Can you work these out from the model? Positions are in its coordinate system, mm. Face numbers are marked on the shaded views. Give positions to 0.01 mm unless a question says otherwise; leave off trailing zeros. Write each loop counter-clockwise with the first axis right and the second up, starting at its lowest first coordinate (ties: lowest second). Pieces come first, ordered by that corner, then holes. Notation, with made-up numbers: M 89.25,-11 L 136.25,-11 A17 cw 136.25,8 Z; hole C 9,55 d9. An arc over 180 degrees is marked long. Use CSV: the item, a comma, the result in double quotes. Start each with the question number.
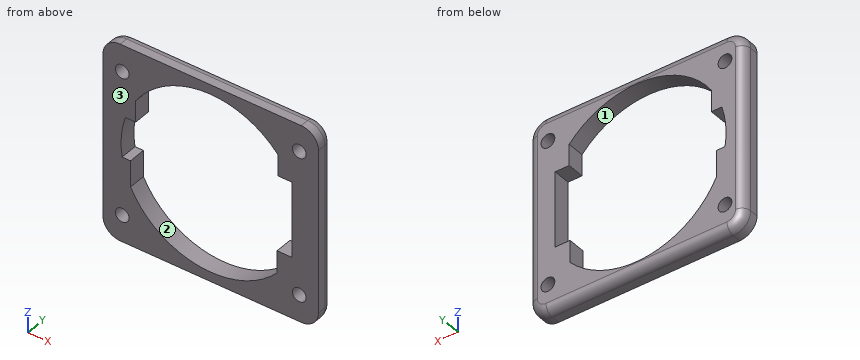
from build123d import *

# Parameters (mm, degrees)
SKETCH1_W           = 31.75
SKETCH1_H           = 29.21
BOSS_EXTRUDE1_DEPTH = 2.54
CUT_EXTRUDE1_DEPTH  = 22.720341848
SKETCH3_W           = 4.064
SKETCH3_H           = 4.263952617
SKETCH3_W_2         = 4.826
SKETCH3_H_2         = 10.541
SKETCH3_W_3         = 5.969
SKETCH3_H_3         = 4.464530762
SKETCH3_W_4         = 6.096
SKETCH3_H_4         = 4.639521707
BOSS_EXTRUDE2_DEPTH = 2.54
FILLET1_R           = 1.27
SKETCH5_R           = 1.016
CUT_EXTRUDE3_DEPTH  = 22.720341848
FILLET2_R           = 2.54


with BuildPart() as part:
    # Sketch1 → Boss-Extrude1 (new body)
    with BuildSketch(Plane(origin=(0, 0, 0), x_dir=(1, 0, 0), z_dir=(0, 1, 0))):
        Rectangle(SKETCH1_W, SKETCH1_H)
    extrude(amount=BOSS_EXTRUDE1_DEPTH)

    # Sketch2 → Cut-Extrude1 (cut, through all)
    with BuildSketch(Plane(origin=(0, 2.54, 0), x_dir=(1, 0, 0), z_dir=(0, 1, 0))):
        with BuildLine():
            Line((11.967686493, 5.588), (11.967686493, -5.588))
            ThreePointArc((11.967686493, -5.588), (-13.208, 0), (11.967686493, 5.588))
        make_face()
    extrude(amount=-CUT_EXTRUDE1_DEPTH, mode=Mode.SUBTRACT)

    # Sketch3 → Boss-Extrude2 (add)
    with BuildSketch(Plane(origin=(0, 2.54, 0), x_dir=(1, 0, 0), z_dir=(0, 1, 0))):
        with Locations((-13.843, 4.163976309)):
            Rectangle(SKETCH3_W, SKETCH3_H)
        with Locations((-13.462, -9.3345)):
            Rectangle(SKETCH3_W_2, SKETCH3_H_2)
        with Locations((12.8905, -7.820265381)):
            Rectangle(SKETCH3_W_3, SKETCH3_H_3)
        with Locations((12.827, 7.907760854)):
            Rectangle(SKETCH3_W_4, SKETCH3_H_4)
    extrude(amount=-BOSS_EXTRUDE2_DEPTH)

    # Fillet1
    fillet1_edges = [part.edges().sort_by_distance(p)[0] for p in [
        (15.875, 2.54, 0),
        (0, 2.54, -14.605),
        (-15.875, 2.54, 0),
        (0, 2.54, 14.605),
    ]]
    fillet(fillet1_edges, radius=FILLET1_R)

    # Sketch5 → Cut-Extrude3 (cut, through all)
    with BuildSketch(Plane.XZ):
        with Locations(Location((13.0429, -10.6553, 0), (0, 0, 270))):
            Circle(SKETCH5_R)
        with Locations(Location((-13.0429, -10.6553, 0), (0, 0, 90))):
            Circle(SKETCH5_R)
        with Locations(Location((-13.0429, 10.6553, 0), (0, 0, 270))):
            Circle(SKETCH5_R)
        with Locations(Location((13.0429, 10.6553, 0), (0, 0, 90))):
            Circle(SKETCH5_R)
    extrude(amount=-CUT_EXTRUDE3_DEPTH, mode=Mode.SUBTRACT)

    # Fillet2
    # the kernel refuses this fillet: 2.54 mm, written as the material it takes off along each edge
    with BuildSketch(Plane(origin=(13.335, 2.54, -12.065), x_dir=(1, 0, 0), z_dir=(0, 0, 1))) as fillet2_piece_1:
        with BuildLine():
            CenterArc((1.27, -1.27), 1.27, 0, 90)
            Line((2.54, -1.27), (2.54, 0))
            Line((2.54, 0), (1.27, 0))
        make_face()
    revolve(axis=Axis((13.335, 2.54, -12.065), (0, 1, 0)), revolution_arc=90, mode=Mode.SUBTRACT)
    with BuildSketch(Plane(origin=(13.335, 2.54, 12.065), x_dir=(0, 0, 1), z_dir=(-1, 0, 0))) as fillet2_piece_2:
        with BuildLine():
            CenterArc((1.27, -1.27), 1.27, 0, 90)
            Line((2.54, -1.27), (2.54, 0))
            Line((2.54, 0), (1.27, 0))
        make_face()
    revolve(axis=Axis((13.335, 2.54, 12.065), (0, 1, 0)), revolution_arc=90, mode=Mode.SUBTRACT)
    with BuildSketch(Plane(origin=(-13.335, 2.54, -12.065), x_dir=(0, 0, -1), z_dir=(1, 0, 0))) as fillet2_piece_3:
        with BuildLine():
            CenterArc((1.27, -1.27), 1.27, 0, 90)
            Line((2.54, -1.27), (2.54, 0))
            Line((2.54, 0), (1.27, 0))
        make_face()
    revolve(axis=Axis((-13.335, 2.54, -12.065), (0, 1, 0)), revolution_arc=90, mode=Mode.SUBTRACT)
    with BuildSketch(Plane(origin=(-13.335, 2.54, 12.065), x_dir=(-1, 0, 0), z_dir=(0, 0, -1))) as fillet2_piece_4:
        with BuildLine():
            CenterArc((1.27, -1.27), 1.27, 0, 90)
            Line((2.54, -1.27), (2.54, 0))
            Line((2.54, 0), (1.27, 0))
        make_face()
    revolve(axis=Axis((-13.335, 2.54, 12.065), (0, 1, 0)), revolution_arc=90, mode=Mode.SUBTRACT)
    with BuildSketch(Plane(origin=(-15.875, -6.35, 14.605), x_dir=(0, 0, -1), z_dir=(0, 1, 0)), Plane(origin=(-15.875, -6.35, -14.605), x_dir=(1, 0, 0), z_dir=(0, 1, 0))) as fillet2_piece_5:
        with BuildLine():
            CenterArc((FILLET2_R, -FILLET2_R), FILLET2_R, 90, 90)
            Line((0, -FILLET2_R), (0, 0))
            Line((0, 0), (FILLET2_R, 0))
        make_face()
    extrude(amount=8.89, mode=Mode.SUBTRACT)
    with BuildSketch(Plane(origin=(15.875, -6.35, -14.605), x_dir=(-1, 0, 0), z_dir=(0, 1, 0)), Plane(origin=(15.875, -6.35, 14.605), x_dir=(0, 0, -1), z_dir=(0, 1, 0))) as fillet2_piece_6:
        with BuildLine():
            CenterArc((FILLET2_R, FILLET2_R), FILLET2_R, 180, 90)
            Line((0, FILLET2_R), (0, 0))
            Line((0, 0), (FILLET2_R, 0))
        make_face()
    extrude(amount=8.89, mode=Mode.SUBTRACT)


solid = part.part
(1) I want a section at B-B (z = -0.75). Write out the boundary of the cut face in (x, y) (3 decimals).
(2) Thinking about a two-plate mould opening in Z: for the marked faces 1, 2 and 3, which applies, released by +Z, released by -Z, zero draft, split by the parting line, or undercut?
(3) I want a section at C-C (z = -10.25). Write out the boundary of the cut face in (x, y) (3 decimals), and give its area (3 significant figures).
(4) I want a section at D-D (y = 0.85). Write out the boundary of the cut face in (x, z) (3 decimals).
(5) I want a section at A-A (x = 11.5). Write out the boundary of the cut face in (y, z) (3 decimals).
(6) Will these pins go through, and if not, where does the flat tip stop? pin 1 Ø1 at (x, y) = (10.5, 2) entering from -Z; pin 2 Ø1.3 at (y, z) = (1.5, 7.5) entering from -X (3 decimals).
(7) Please list where these lines run through material, in increasing order: L1, parallel to Z at x = 12.5, y = 2.4; L2, parallel to X at y = 2.15, z = 10.5; L3, parallel to X at y = 0.1, z = -4 (3 decimals). Write a range as [from, to].
Geometry results:
1,outline,"M -15.875,0 L -13.187,0 L -13.187,2.54 L -14.605,2.54 A1.27 ccw -15.875,1.27 Z; M 11.968,0 L 15.875,0 L 15.875,1.27 A1.27 ccw 14.605,2.54 L 11.968,2.54 Z"
2,face 1,"undercut"
2,face 2,"undercut"
2,face 3,"zero draft"
3,outline,"M -15.875,0 L -13.975,0 L -13.975,2.54 L -14.605,2.54 A1.27 ccw -15.875,1.27 Z; M -12.111,0 L -8.33,0 L -8.33,2.54 L -12.111,2.54 Z; M 8.33,0 L 12.111,0 L 12.111,2.54 L 8.33,2.54 Z; M 13.975,0 L 15.875,0 L 15.875,1.27 A1.27 ccw 14.605,2.54 L 13.975,2.54 Z"
3,area,"28.2 mm2"
4,outline,"M -15.875,-12.065 A2.54 ccw -13.335,-14.605 L 13.335,-14.605 A2.54 ccw 15.875,-12.065 L 15.875,12.065 A2.54 ccw 13.335,14.605 L -13.335,14.605 A2.54 ccw -15.875,12.065 Z; hole C -13.043,-10.655 d2.032; hole C -13.043,10.655 d2.032; hole M -13.051,-2.032 L -11.811,-2.032 L -11.811,-5.912 A13.208 ccw 9.779,-8.878 L 9.779,-5.588 L 11.968,-5.588 L 11.968,5.588 L 9.906,5.588 L 9.906,8.736 A13.208 ccw -11.049,7.237 L -11.049,4.064 L -12.567,4.064 A13.208 ccw Z; hole C 13.043,-10.655 d2.032; hole C 13.043,10.655 d2.032"
5,outline,"M 0,-14.605 L 1.27,-14.605 A1.27 ccw 2.54,-13.335 L 2.54,-5.588 L 0,-5.588 Z; M 0,5.588 L 2.54,5.588 L 2.54,13.335 A1.27 ccw 1.27,14.605 L 0,14.605 Z"
6,pin 1,"stops at z = -14.58"
6,pin 2,"stops at x = -15.875"
7,L1,"z = [-13.91, -11.51], [-9.8, 9.8], [11.51, 13.91]"
7,L2,"x = [-15.52, -14.05], [-12.04, -8.01], [8.01, 12.04], [14.05, 15.52]"
7,L3,"x = [-15.875, -11.811], [11.968, 15.875]"
